Design review of the part built by this model. Coordinates are the model's own, in mm. Coordinates: 2 decimals unless noted, no trailing zeros. Write each loop counter-clockwise with the first axis right and the second up, starting at its lowest first coordinate (ties: lowest second). Pieces come first, ordered by that corner, then holes. Notation, with made-up numbers: (47, 14) - (51, 14) arc R8 cw to (51, 21) - close; hole circle Ø5 at (35.25, 42.5). An arc over 180 degrees is marked (long way). One line per item, written item: value.
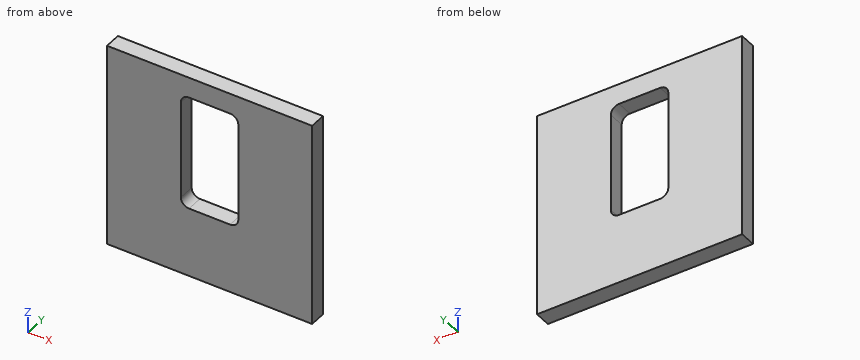
from build123d import *

# Parameters (mm, degrees)
SKETCH1_W           = 25
SKETCH1_H           = 25
BOSS_EXTRUDE1_DEPTH = 1
CUT_EXTRUDE1_REACH  = 19.79
SKETCH2_W           = 7
SKETCH2_H           = 14
FILLET1_R           = 1


with BuildPart() as part:
    # Sketch1 → Boss-Extrude1 (new, symmetric)
    with BuildSketch(Plane(origin=(0, 0, 0), x_dir=(1, 0, 0), z_dir=(0, 1, 0))):
        Rectangle(SKETCH1_W, SKETCH1_H)
    extrude(amount=BOSS_EXTRUDE1_DEPTH, both=True)

    # Sketch2 → Cut-Extrude1 (cut, up to next)
    with BuildSketch(Plane(origin=(0, 1, 0), x_dir=(1, 0, 0), z_dir=(0, 1, 0)), mode=Mode.PRIVATE) as cut_extrude1_sk1:
        with Locations((0, -3)):
            Rectangle(SKETCH2_W, SKETCH2_H)
    cut_extrude1_tool1 = extrude(cut_extrude1_sk1.sketch, amount=-CUT_EXTRUDE1_REACH, mode=Mode.PRIVATE) & part.part
    add(cut_extrude1_tool1.solids().sort_by_distance((0, 1, 3))[0], mode=Mode.SUBTRACT)

    # Fillet1
    fillet1_edges = [part.edges().sort_by_distance(p)[0] for p in [
        (-3.5, 0, 10),
        (-3.5, 0, -4),
        (3.5, 0, -4),
        (3.5, 0, 10),
    ]]
    fillet(fillet1_edges, radius=FILLET1_R)


solid = part.part
1. Consider section A-A, the plane x = -1.5. Write out the cut boundary in (y, z).
Answer block:
outline: (-1, -12.5) - (1, -12.5) - (1, -4) - (-1, -4) - close; (-1, 10) - (1, 10) - (1, 12.5) - (-1, 12.5) - close
2. Wall thickness on line 1 along Z through (x, y) = (2.5, 0.45); line 2 along X through (y, z) = (0.3, 2.5); line 3 along Z through (x, y) = (-3.25, 0.1): over which ranges is each line inside the solid? List them lowest first.
Answer block:
line 1: z = -12.5 to -4, 10 to 12.5
line 2: x = -12.5 to -3.5, 3.5 to 12.5
line 3: z = -12.5 to -3.66, 9.66 to 12.5
3. Consider section B-B, the plane z = 6.75. Write out the cut boundary in (x, y), then the cut area to 3 significant figures.
Answer block:
outline: (-12.5, -1) - (-3.5, -1) - (-3.5, 1) - (-12.5, 1) - close; (3.5, -1) - (12.5, -1) - (12.5, 1) - (3.5, 1) - close
area: 36.0 mm^2
4. Consider section C-C, the plane y = -0.35. Write out the cut boundary in (x, z), then the cut area to 3 significant figures.
Answer block:
outline: (-12.5, -12.5) - (12.5, -12.5) - (12.5, 12.5) - (-12.5, 12.5) - close; hole (-3.5, -3) arc R1 ccw to (-2.5, -4) - (2.5, -4) arc R1 ccw to (3.5, -3) - (3.5, 9) arc R1 ccw to (2.5, 10) - (-2.5, 10) arc R1 ccw to (-3.5, 9) - close
area: 528 mm^2
